Here's the drawing with two shaded views (mm, measured from the low corner). I have some questions. A direction names the side the tool comes from. Coordinates: 2 decimals unless noted, no trailing zeros. Write each loop counter-clockwise with the first axis right and the second up, starting at its lowest first coordinate (ties: lowest second). Pieces come first, ordered by that corner, then holes. Notation, with made-up numbers: (29, -14.75) -> (42, -14.75) arc R22 ccw to (42, -2.75) -> close; hole circle Ø1 at (88.25, 68.25). An arc over 180 degrees is marked (long way). Put each result on its own line as item: value. Start each with the question number.
Item 1: I want a section at C-C, the plane z = 0.55. List the corners of the cut face in (x, y) for me, then the cut area to 3 significant figures.
Item 2: For pin 1 (2 mm diameter, centred on y = 5, z = 2, fed in from +X), with a flat end and sliding along its axis, tell me the tip position at first contact or that it passes through.
Item 3: On a 3-axis mill with a long thin cutter (end or side, diameter ignored), from which of +Z, -Z, +X, -X, +Y, -Y can I reach the whole of each face in a straight line? I mean the marked faces 1 and 2. Say none if no direction works.
Item 4: I want a section at D-D, the plane y = 0.6. List the corners of the cut face in (x, z) for me.
Item 5: If we mould it in two halves opening along Y, with no side actions, what happens to the marked faces 3, 4 and 5? For each: released by +Y, released by -Y, zero draft, split by the parting line, or undercut.
Item 6: I need wall thicknesses on line 1 (Y direction, x = 3, z = 3.3); line 2 (Y direction, x = 3, z = 2.3); line 3 (Z direction, x = 1.2, y = 0.7). Which ranges of each line are inside material? Lowest first, please. Write a range as [from, to].
Item 7: I want a section at A-A, the plane y = 3. List the corners of the cut face in (x, z) for me.
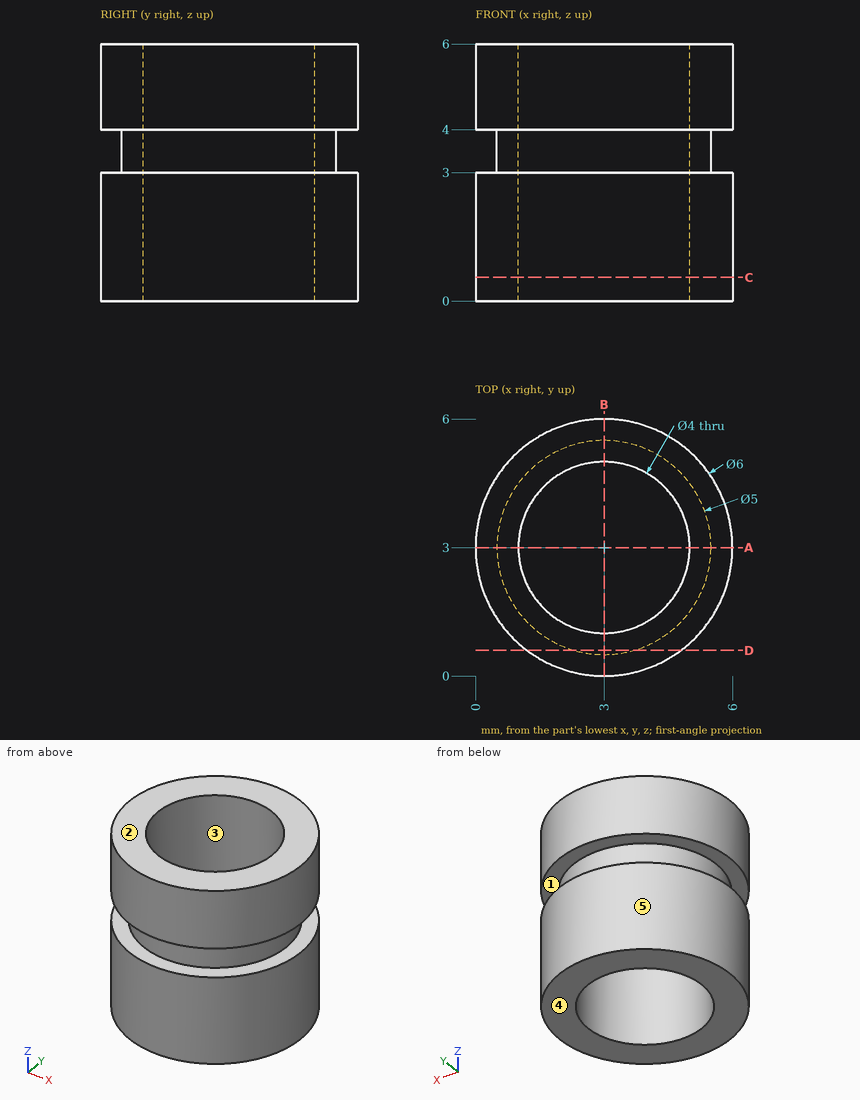
Calculated:
1. outline: circle Ø6 at (3, 3); hole circle Ø4 at (3, 3)
1. area: 15.7 mm2
2. pin 1: stops at x = 5.83
3. face 1: none
3. face 2: +Z, +X, -X, +Y, -Y
4. outline: (1.2, 0) -> (4.8, 0) -> (4.8, 3) -> (3.7, 3) -> (3.7, 4) -> (4.8, 4) -> (4.8, 6) -> (1.2, 6) -> (1.2, 4) -> (2.3, 4) -> (2.3, 3) -> (1.2, 3) -> close
5. face 3: undercut
5. face 4: zero draft
5. face 5: split by the parting line
6. line 1: y = [0.5, 1], [5, 5.5]
6. line 2: y = [0, 1], [5, 6]
6. line 3: z = [0, 3], [4, 6]
7. outline: (0, 0) -> (1, 0) -> (1, 6) -> (0, 6) -> (0, 4) -> (0.5, 4) -> (0.5, 3) -> (0, 3) -> close; (5, 0) -> (6, 0) -> (6, 3) -> (5.5, 3) -> (5.5, 4) -> (6, 4) -> (6, 6) -> (5, 6) -> close
